Geometry check sheet. Reference: the model listing, model coordinates, mm. A direction names the side the tool comes from. Give positions to 0.01 mm unless a question says otherwise; leave off trailing zeros. Write each loop counter-clockwise with the first axis right and the second up, starting at its lowest first coordinate (ties: lowest second). Pieces come first, ordered by that corner, then holes. Notation, with made-up numbers: (16.25, -17.5) - (55.25, -17.5) arc R22 cw to (55.25, 0.5) - close; hole circle Ø6 at (88.5, -27.75). An arc over 180 degrees is marked (long way). Use a Markdown table: item, result.
```python
from build123d import *

# Parameters (mm, degrees)
SKETCH_W     = 50
SKETCH_H     = 56
SKETCH_R     = 1.375
SKETCH_R_2   = 17.5
PAD_DEPTH    = 2
SKETCH001_R  = 3
PAD001_DEPTH = 24.9
SKETCH002_R  = 1.25
PAD002_DEPTH = 26.9


with BuildPart() as part:
    # Sketch → Pad (new body)
    with BuildSketch(Plane.XY):
        Rectangle(SKETCH_W, SKETCH_H)
        with Locations((-22, 25)):
            Circle(SKETCH_R, mode=Mode.SUBTRACT)
        with Locations((13.5, 25)):
            Circle(SKETCH_R, mode=Mode.SUBTRACT)
        with Locations((-22, -25)):
            Circle(SKETCH_R, mode=Mode.SUBTRACT)
        with Locations((13.5, -25)):
            Circle(SKETCH_R, mode=Mode.SUBTRACT)
        Circle(SKETCH_R_2, mode=Mode.SUBTRACT)
    extrude(amount=PAD_DEPTH)

    # Sketch001 → Pad001 (join)
    with BuildSketch(Plane.XY):
        with Locations((-22, 17)):
            Circle(SKETCH001_R)
        with Locations((22, 17)):
            Circle(SKETCH001_R)
        with Locations((22, -17)):
            Circle(SKETCH001_R)
        with Locations((-22, -17)):
            Circle(SKETCH001_R)
    extrude(amount=PAD001_DEPTH)

    # Sketch002 → Pad002 (join)
    with BuildSketch(Plane.XY):
        with Locations((-22, 17)):
            Circle(SKETCH002_R)
        with Locations((22, 17)):
            Circle(SKETCH002_R)
        with Locations((22, -17)):
            Circle(SKETCH002_R)
        with Locations((-22, -17)):
            Circle(SKETCH002_R)
    extrude(amount=PAD002_DEPTH)


solid = part.part
```
1) Section check D-D on x = 22. Record the boundary of the cut face in (y, z), then the cut area to 3 significant figures.
Working result:
| item | result |
|---|---|
| outline | (-28, 0) - (28, 0) - (28, 2) - (20, 2) - (20, 24.9) - (18.25, 24.9) - (18.25, 26.9) - (15.75, 26.9) - (15.75, 24.9) - (14, 24.9) - (14, 2) - (-14, 2) - (-14, 24.9) - (-15.75, 24.9) - (-15.75, 26.9) - (-18.25, 26.9) - (-18.25, 24.9) - (-20, 24.9) - (-20, 2) - (-28, 2) - close |
| area | 397 mm² |
2) Section check B-B on y = 0. Record the boundary of the cut face in (x, z).
Working result:
| item | result |
|---|---|
| outline | (-25, 0) - (-17.5, 0) - (-17.5, 2) - (-25, 2) - close; (17.5, 0) - (25, 0) - (25, 2) - (17.5, 2) - close |
3) Section check C-C on x = 4. Record the boundary of the cut face in (y, z), then the cut area to 3 significant figures.
Working result:
| item | result |
|---|---|
| outline | (-28, 0) - (-17.04, 0) - (-17.04, 2) - (-28, 2) - close; (17.04, 0) - (28, 0) - (28, 2) - (17.04, 2) - close |
| area | 43.9 mm² |
4) Set-up check for faces 1 (the flat face through (23, 16, 24.9)), 2 (the cylindrical face through (12.487, 25.929, 0.986)): record each of +Z, -Z, +X, -X, +Y, -Y from which the full face is reachable in a straight line by a thin tool's end or side.
Working result:
| item | result |
|---|---|
| face 1 | +Z |
| face 2 | +Z, -Z |
5) Material ranges on L1, parallel to Y at x = 0, z = 0.8; L2, parallel to Y at x = 13.5, z = 1.5 (3 decimals); L3, parallel to Z at x = -15, y = 10, recorded low to high. Write a range as from..to.
Working result:
| item | result |
|---|---|
| L1 | y = -28..-17.5, 17.5..28 |
| L2 | y = -28..-26.375, -23.625..-11.136, 11.136..23.625, 26.375..28 |
| L3 | z = 0..2 |
6) Depth check by flat-ended pin: P1, Ø3.5, axis at x = -22, y = 25, coming from the +Z side; P2, Ø12, axis at x = -17, y = 18, coming from the +Z side; P3, Ø5, axis at x = -13.5, y = 5.5, coming from the +Z side; P4, Ø1.5, axis at y = -13.5, z = 13, coming from the -X side. Enter the tip coordinate at first touch or a pass-through.
Working result:
| item | result |
|---|---|
| P1 | stops at z = 2 |
| P2 | stops at z = 26.9 |
| P3 | passes through |
| P4 | stops at x = -23.2 |
7) Mould release check, pull along X, two halves, no side actions. Record for faces 3 (the flat face through (-21, 16, 24.9)), 4 (the flat face through (25, 0, 1)), 5 (the flat face through (-22, 17, 26.9)): pulls with the +X half, pulls with the -X half, needs draft (parallel to the pull), parting line crosses it, or undercut.
Working result:
| item | result |
|---|---|
| face 3 | undercut |
| face 4 | pulls with the +X half |
| face 5 | needs draft |
8) Section check A-A on y = -25. Record the boundary of the cut face in (x, z) (3 decimals), then the cut area to 3 significant figures.
Working result:
| item | result |
|---|---|
| outline | (-25, 0) - (-23.375, 0) - (-23.375, 2) - (-25, 2) - close; (-20.625, 0) - (12.125, 0) - (12.125, 2) - (-20.625, 2) - close; (14.875, 0) - (25, 0) - (25, 2) - (14.875, 2) - close |
| area | 89.0 mm² |
